from build123d import *

# Parameters (mm, degrees)
F2_R     = 2
F3_DEPTH = 25.4
F4_R     = 6.5
F5_DEPTH = 9


with BuildPart() as f1:
    # F0 (on Top) → F1 (revolve)
    with BuildSketch(Plane.XY):
        with BuildLine():
            Line((0, -58), (0, -68))
            ThreePointArc((0, -68), (3.242526, -73.600747), (4.207879, -80))
            Line((4.207879, -80), (7, -80))
            Line((7, -80), (7, -58))
            Line((7, -58), (0, -58))
        make_face()
    revolve(axis=Axis((7, -68.5, 0), (0, 1, 0)))

    # F2 (on Right) → F3 (cut)
    with BuildSketch(Plane.YZ):
        with Locations((-76.524546, -0.129668)):
            Circle(F2_R)
    extrude(amount=F3_DEPTH, mode=Mode.SUBTRACT)

    # F4 (on face) → F5 (cut)
    with BuildSketch(Plane(origin=(0, -58, 0), x_dir=(-1, 0, 0), z_dir=(0, 1, 0))):
        with Locations((-7, 0)):
            Circle(F4_R)
    extrude(amount=-F5_DEPTH, mode=Mode.SUBTRACT)


solid = f1.part
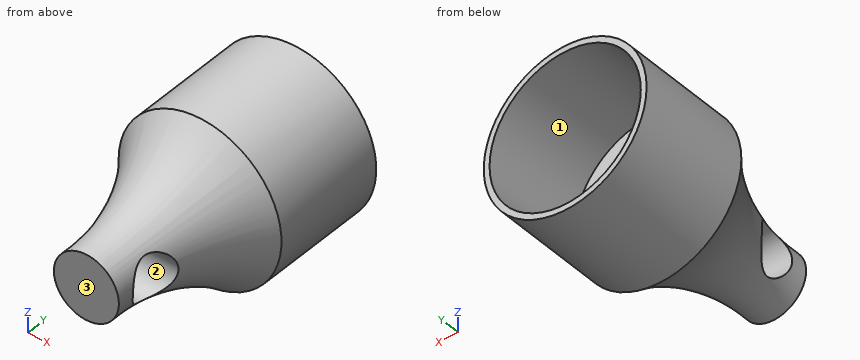
The model under review builds one solid part; all positions refer to its coordinate system, in mm. Face numbers are marked on the shaded views. Give positions to 0.01 mm unless a question says otherwise; leave off trailing zeros. Write each loop counter-clockwise with the first axis right and the second up, starting at its lowest first coordinate (ties: lowest second). Pieces come first, ordered by that corner, then holes.
1. Draft analysis for pull direction Y (two halves, no side actions). For the marked faces 1, 2 and 3, state which applies: +Y half, -Y half, draft (parallel to the pull), parting line (faces both ways), or undercut.
2. Add section A-A, the plane x = 7. Write out the cut boundary in (y, z), plus the area to 3 significant figures.
3. Add section B-B, the plane y = -62.5. Write out the cut boundary in (x, z).
4. Add section D-D, the plane y = -76.5. Write out the cut boundary in (x, z).
5. For P1, Ø8, axis at x = 10, y = -76, coming from the -Z side; P2, Ø3.5, axis at y = -76.52, z = -0.13, coming from the -X side; P3, Ø1, axis at x = 11.5, y = -60.5, coming from the +Z side; P4, Ø6, axis at y = -70.5, z = 2.5, coming from the +X side, all flat-tipped, find the tip position at first contact; note any pin that passes through.
6. Wall thickness on L1, parallel to Z at x = 7, y = -61.75; L2, parallel to Y at x = 5.25, z = 0; L3, parallel to Y at x = 8, z = 1: over which ranges is each line inside the solid? List them lowest first.
7. Add section C-C, the plane y = -69. Write out the cut boundary in (x, z), plus the area to 3 significant figures.
Worked answers:
1. face 1: draft
1. face 2: undercut
1. face 3: -Y half
2. outline: (-80, -2.79) arc R17.36 cw to (-68, -7) - (-58, -7) - (-58, -6.5) - (-67, -6.5) - (-67, 6.5) - (-58, 6.5) - (-58, 7) - (-68, 7) arc R17.36 cw to (-80, 2.79) - close; hole circle Ø4 at (-76.52, -0.13)
2. area: 107 mm2
3. outline: circle Ø14 at (7, 0); hole circle Ø13 at (7, 0)
4. outline: (4.64, 1.87) - (9.36, 1.87) arc R3.01 ccw to start; (4.87, -2.13) arc R3.01 ccw to (9.13, -2.13) - close
5. P1: stops at z = -4.05
5. P2: passes through
5. P3: stops at z = 5.74
5. P4: stops at x = 13.95
6. L1: z = -7 to -6.5, 6.5 to 7
6. L2: y = -80 to -78.52, -74.53 to -67
6. L3: y = -80 to -78.17, -74.87 to -67
7. outline: circle Ø12.4 at (7, 0)
7. area: 121 mm2
